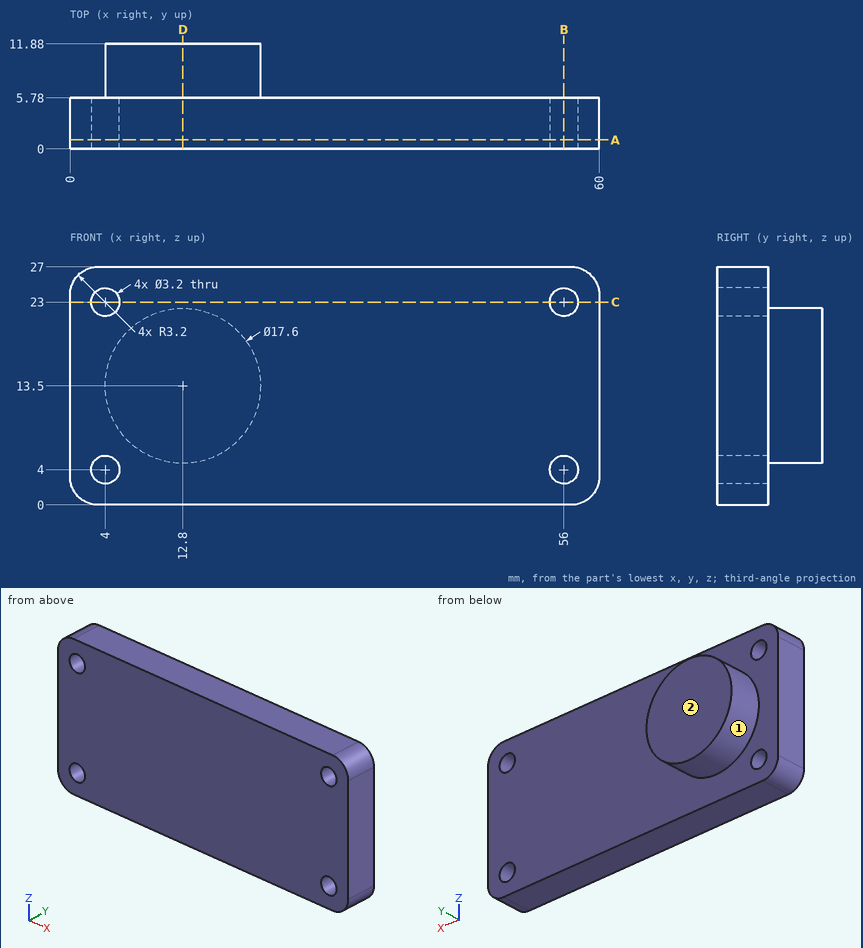
Could you check a few things on this drawing? It's one solid part, dimensions in mm from its lowest x, y, z. A direction names the side the tool comes from. Coordinates: 2 decimals unless noted, no trailing zeros. Order: outer loops, then holes, each group sorted by start corner. A loop starts at its lowest first (then second) coordinate and runs counter-clockwise, first axis right, second up. Notation, with made-up numbers: M 16.5,33.25 L 63.5,33.25 A4 ccw 63.5,40.25 Z; hole C -8.75,48.25 d4. An arc over 180 degrees is marked long. Use one line per item in the form item = value. Start each with the question number.
1. Suppose I cut it at B-B on x = 56. Write out the boundary of the cut face in (y, z).
2. Suppose I cut it at A-A on y = 1. Write out the boundary of the cut face in (x, z), then the cut area to 3 significant figures.
3. On a 3-axis mill with a long thin cutter (end or side, diameter ignored), from which of +Z, -Z, +X, -X, +Y, -Y can I reach the whole of each face in a straight line? I mean the marked faces 1 and 2. Say none if no direction works.
4. Suppose I cut it at D-D on x = 12.8. Write out the boundary of the cut face in (y, z), then the cut area to 3 significant figures.
5. Please list where these lines run through material, in increasing order: line 1 (X direction, y = 1.7, z = 23); line 2 (Z direction, x = 4, y = 3); line 3 (X direction, y = 2, z = 2.75).
6. Suppose I cut it at C-C on z = 23. Write out the boundary of the cut face in (x, y).
7. For pin 1 (1.9 mm diameter, centred on x = 4, z = 4, fed in from -Y); pin 2 (8 mm diameter, centred on x = 37, z = 20, fed in from +Y), each with a flat end and sliding along its axis, tell me the tip position at first contact or that it passes through.
Geometry says:
q1.outline = M 0,0 L 5.78,0 L 5.78,2.4 L 0,2.4 Z; M 0,5.6 L 5.78,5.6 L 5.78,21.4 L 0,21.4 Z; M 0,24.6 L 5.78,24.6 L 5.78,27 L 0,27 Z
q2.outline = M 0,3.2 A3.2 ccw 3.2,0 L 56.8,0 A3.2 ccw 60,3.2 L 60,23.8 A3.2 ccw 56.8,27 L 3.2,27 A3.2 ccw 0,23.8 Z; hole C 4,4 d3.2; hole C 4,23 d3.2; hole C 56,4 d3.2; hole C 56,23 d3.2
q2.area = 1,580 mm^2
q3.face_1 = +Y
q3.face_2 = +Z, -Z, +X, -X, +Y
q4.outline = M 0,0 L 5.78,0 L 5.78,4.7 L 11.88,4.7 L 11.88,22.3 L 5.78,22.3 L 5.78,27 L 0,27 Z
q4.area = 263 mm^2
q5.line_1 = 0 to 2.4, 5.6 to 54.4, 57.6 to 60
q5.line_2 = 0 to 2.4, 5.6 to 21.4, 24.6 to 27
q5.line_3 = 0.03 to 3, 5 to 55, 57 to 59.97
q6.outline = M 0,0 L 2.4,0 L 2.4,5.78 L 0,5.78 Z; M 5.6,0 L 54.4,0 L 54.4,5.78 L 5.6,5.78 Z; M 57.6,0 L 60,0 L 60,5.78 L 57.6,5.78 Z
q7.pin_1 = through
q7.pin_2 = 5.78
